Geometry: final body of the model. Coordinates: model frame, mm. Face numbers are marked on the shaded views. A direction names the side the tool comes from. Give positions to 0.01 mm unless a question says otherwise; leave off trailing zeros. Write each loop counter-clockwise with the first axis right and the second up, starting at its lowest first coordinate (ties: lowest second). Pieces come first, ordered by that corner, then holes.
Q1. Section A-A (y = -35). Return the cut outline in (x, z).
Q2. Reachability of the marked faces 4, 5, 6 and 7 from +Z, -Z, +X, -X, +Y, -Y: full face, straight path, thin tool, end or side. Return the list, or none.
Q3. Line query: line 1 (Y direction, x = 2.5, z = 56); line 2 (X direction, y = -25.5, z = 76.5); line 3 (Z direction, x = -65, y = -38.5). Output: solid intervals per line, ascending.
Q4. Section B-B (x = -26). Return the cut outline in (y, z).
Q5. Pin query (flat end, axial travel): pin 1 Ø3 at (y, z) = (-7, 67) entering from -X; pin 2 Ø12 at (x, z) = (51, 34.5) entering from +Y; pin 3 Ø3 at (x, y) = (-20.5, 12) entering from -Z. Return the tip coordinate at first contact, or that it passes through.
Q6. Mould query, pull axis Y, two halves, no side actions, for the marked faces 1, 2 and 3. Classes: +Y half, -Y half, draft (parallel to the pull), parting line (faces both ways), or undercut.
Q7. Section C-C (z = 102.5). Return the cut outline in (x, y).
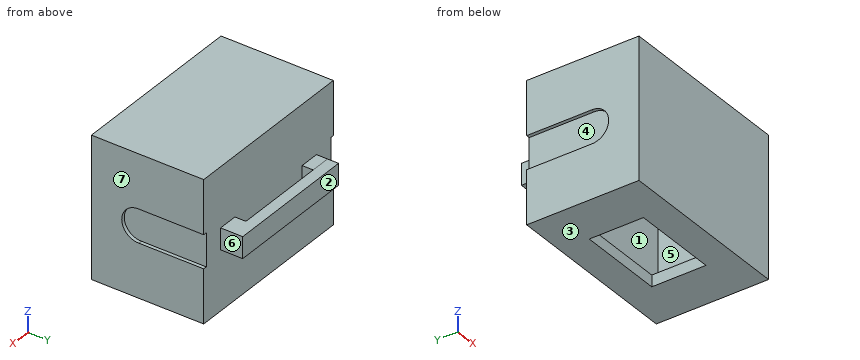
from build123d import *

# Parameters (mm, degrees)
SKETCH2_W           = 162.951605996
SKETCH2_H           = 101.6
BOSS_EXTRUDE1_DEPTH = 127
SKETCH6_W           = 150.072334712
SKETCH6_H           = 88.9
CUT_EXTRUDE1_DEPTH  = 114.3
SKETCH14_W          = 29.9974
SKETCH14_H          = 58.598040667
CUT_EXTRUDE2_DEPTH  = 3.22
SKETCH15_R          = 15
CUT_EXTRUDE3_DEPTH  = 3.22
SKETCH17_W          = 29.9974
SKETCH17_H          = 58.598040667
CUT_EXTRUDE4_DEPTH  = 3.22
CUT_EXTRUDE5_START  = -3.22
SKETCH18_R          = 15
CUT_EXTRUDE5_DEPTH  = 3.22
SKETCH19_W          = 18
SKETCH19_H          = 19.33286688
SKETCH19_H_2        = 19.332866873
BOSS_EXTRUDE2_DEPTH = 10
SKETCH20_W          = 120.511605996
SKETCH20_H          = 19.329300313
BOSS_EXTRUDE3_DEPTH = 10
SKETCH28_W          = 150.072334712
SKETCH28_H          = 88.9
BOSS_EXTRUDE5_DEPTH = 10.33404711
SKETCH29_W          = 78.5832061
SKETCH29_H          = 48.996471626
CUT_EXTRUDE6_DEPTH  = 10.33404711


with BuildPart() as part:
    # Sketch2 → Boss-Extrude1 (new body)
    with BuildSketch(Plane.XY):
        Rectangle(SKETCH2_W, SKETCH2_H)
    extrude(amount=BOSS_EXTRUDE1_DEPTH)

    # Sketch6 → Cut-Extrude1 (cut)
    with BuildSketch(Plane.XY):
        Rectangle(SKETCH6_W, SKETCH6_H)
    extrude(amount=CUT_EXTRUDE1_DEPTH, mode=Mode.SUBTRACT)

    # Sketch14 → Cut-Extrude2 (cut)
    with BuildSketch(Plane.ZY.offset(81.475802998)):
        with Locations((63.5013, 21.500979667)):
            Rectangle(SKETCH14_W, SKETCH14_H)
    extrude(amount=-CUT_EXTRUDE2_DEPTH, mode=Mode.SUBTRACT)

    # Sketch15 → Cut-Extrude3 (cut)
    with BuildSketch(Plane.ZY.offset(81.475802998)):
        with Locations((63.5013, -8.386572038)):
            Circle(SKETCH15_R)
    extrude(amount=-CUT_EXTRUDE3_DEPTH, mode=Mode.SUBTRACT)

    # Sketch17 → Cut-Extrude4 (cut)
    with BuildSketch(Plane(origin=(81.475802998, 0, 0), x_dir=(0, 0, -1), z_dir=(1, 0, 0))):
        with Locations((-63.5013, 21.500979667)):
            Rectangle(SKETCH17_W, SKETCH17_H)
    extrude(amount=-CUT_EXTRUDE4_DEPTH, mode=Mode.SUBTRACT)

    # Sketch18 → Cut-Extrude5 (cut)
    with BuildSketch(Plane(origin=(81.475802998, 0, 0), x_dir=(0, 0, -1), z_dir=(1, 0, 0)).offset(CUT_EXTRUDE5_START)):
        with Locations((-63.5013, -8.386572038)):
            Circle(SKETCH18_R)
    extrude(amount=CUT_EXTRUDE5_DEPTH, mode=Mode.SUBTRACT)

    # Sketch19 → Boss-Extrude2 (add)
    with BuildSketch(Plane(origin=(0, 50.8, 0), x_dir=(1, 0, 0), z_dir=(0, 1, 0))):
        with Locations((-51.255802998, -63.5)):
            Rectangle(SKETCH19_W, SKETCH19_H)
        with Locations((51.255802998, -63.496433436)):
            Rectangle(SKETCH19_W, SKETCH19_H_2)
    extrude(amount=BOSS_EXTRUDE2_DEPTH)

    # Sketch20 → Boss-Extrude3 (add)
    with BuildSketch(Plane(origin=(0, 60.8, 0), x_dir=(1, 0, 0), z_dir=(0, 1, 0))):
        with Locations((0, -63.498216716)):
            Rectangle(SKETCH20_W, SKETCH20_H)
    extrude(amount=BOSS_EXTRUDE3_DEPTH)

    # Sketch28 → Boss-Extrude5 (add)
    with BuildSketch(Plane.XY):
        Rectangle(SKETCH28_W, SKETCH28_H)
    extrude(amount=BOSS_EXTRUDE5_DEPTH)

    # Sketch29 → Cut-Extrude6 (cut)
    with BuildSketch(Plane.XY):
        Rectangle(SKETCH29_W, SKETCH29_H)
    extrude(amount=CUT_EXTRUDE6_DEPTH, mode=Mode.SUBTRACT)


solid = part.part
Computed:
1. outline: (-81.48, 0) - (81.48, 0) - (81.48, 127) - (-81.48, 127) - close; hole (-75.04, 10.33) - (75.04, 10.33) - (75.04, 114.3) - (-75.04, 114.3) - close
2. face 4: -X, +Y
2. face 5: none
2. face 6: +Z, -Z, +X, +Y
2. face 7: +Z, -Z, +X, +Y, -Y
3. line 1: y = -50.8 to -44.45, 44.45 to 50.8, 60.8 to 70.8
3. line 2: x = -81.48 to -75.04, 75.04 to 81.48
3. line 3: z = 0 to 10.33, 114.3 to 127
4. outline: (-50.8, 0) - (-24.5, 0) - (-24.5, 10.33) - (-44.45, 10.33) - (-44.45, 114.3) - (44.45, 114.3) - (44.45, 10.33) - (24.5, 10.33) - (24.5, 0) - (50.8, 0) - (50.8, 127) - (-50.8, 127) - close; (60.8, 53.83) - (70.8, 53.83) - (70.8, 73.16) - (60.8, 73.16) - close
5. pin 1: stops at x = -78.26
5. pin 2: stops at y = 50.8
5. pin 3: stops at z = 114.3
6. face 1: undercut
6. face 2: +Y half
6. face 3: draft
7. outline: (-81.48, -50.8) - (81.48, -50.8) - (81.48, 50.8) - (-81.48, 50.8) - close; hole (-75.04, -44.45) - (75.04, -44.45) - (75.04, 44.45) - (-75.04, 44.45) - close
